The figure shows three views and two pictorial views of one solid part (mm, origin at its lowest corner). Answer the questions. Coordinates: 2 decimals unless noted, no trailing zeros. Loops run counter-clockwise (first coordinate to the right, second up) from the corner with the lowest first, then second, coordinate; pieces in that order, holes last. Notation, with made-up numbers: M 17,-11 L 47,-11 A27 cw 47,21 Z; hole C 9.25,6 d3. An arc over 180 degrees is marked long. Answer in a Markdown table with one row per item. Add a question column.
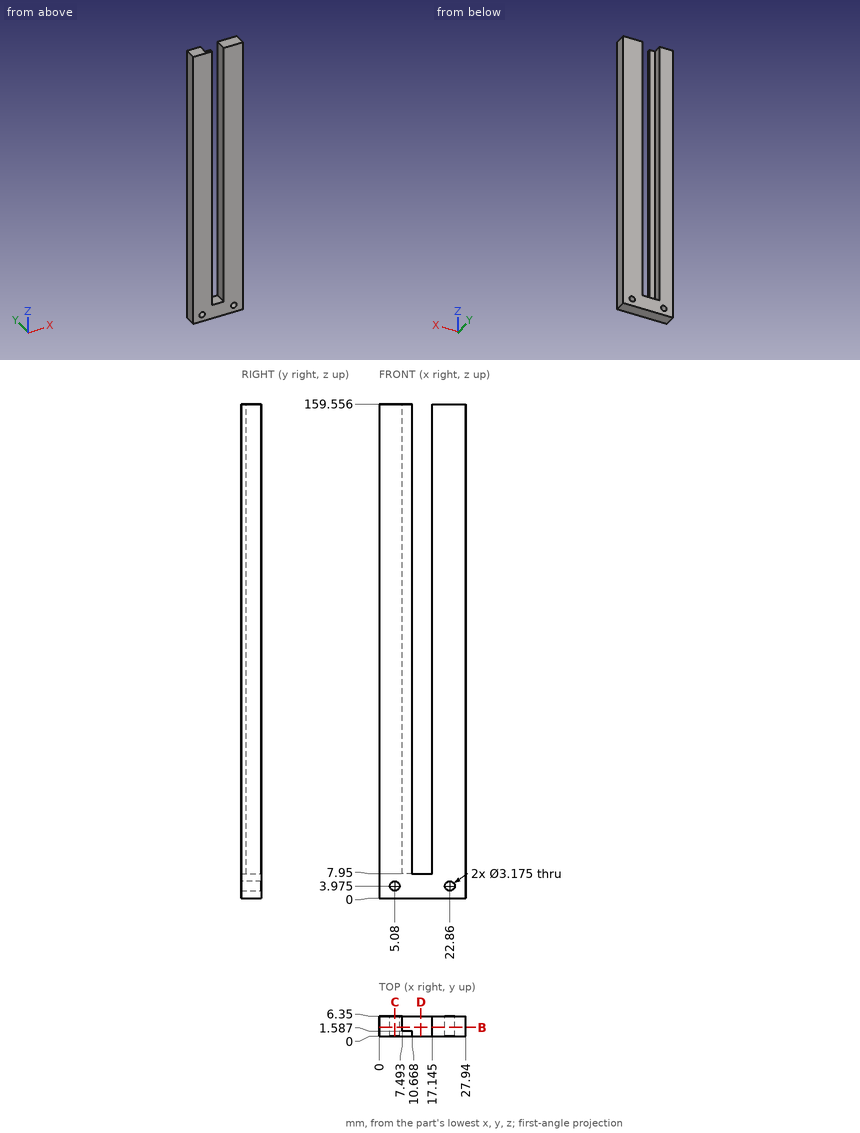
(1) This flat-tipped pin is pushed along its axis until it touches: pin 1 (2.5 mm diameter, centred on x = 9, z = 50.5, fed in from +Y). Where does it stop, or does it pass through?
(2) A cutting plane is placed at B-B (y = 2.75). State how many separate pieces and enclosed holes the cut face has, plus the area to 3 significant figures.
(3) Straight lines are drawn through the part: line 1 (X direction, y = 3.5, z = 114.5) (1 decimal); line 2 (X direction, y = 0.75, z = 48.5) (1 decimal); line 3 (Z direction, x = 24, y = 2) (1 decimal). For each, find the intervals that lie inside material, in ascending order.
(4) A cutting plane is placed at D-D (x = 13.5). Give the vertices of the cut face in (y, z), plus the area to 3 significant figures.
(5) A cutting plane is placed at C-C (x = 5.08). Give the vertices of the cut face in (y, z).
Solved:
| question | item | result |
|---|---|---|
| 1 | pin 1 | stops at y = 1.59 |
| 2 | separate pieces | 1 |
| 2 | enclosed holes | 2 |
| 2 | area | 2,980 mm² |
| 3 | line 1 | x = 0 to 7.5, 17.1 to 27.9 |
| 3 | line 2 | x = 0 to 10.7, 17.1 to 27.9 |
| 3 | line 3 | z = 0 to 2.9, 5.1 to 159.6 |
| 4 | outline | M 0,0 L 6.35,0 L 6.35,7.95 L 0,7.95 Z |
| 4 | area | 50.5 mm² |
| 5 | outline | M 0,0 L 6.35,0 L 6.35,2.39 L 0,2.39 Z; M 0,5.56 L 6.35,5.56 L 6.35,159.56 L 0,159.56 Z |
